Model file for the job. Use its own axes, mm. Face numbers are marked on the shaded views. A direction names the side the tool comes from. Coordinates: 2 decimals unless noted, no trailing zeros. Write each loop counter-clockwise with the first axis right and the second up, starting at its lowest first coordinate (ties: lowest second). Pieces come first, ordered by that corner, then holes. Notation, with made-up numbers: M -18,-9.5 L 0,-9.5 A27 ccw 0,28.5 Z; hole C -36.5,-13 d9. An arc over 180 degrees is marked long. One line per question, with ' | ' between items. Start each with the question number.
(1) Cut at A-A (x = -1415). Write the cut outline in (y, z).
(2) Cut at D-D (x = -1448.5). Write the cut outline in (y, z).
(3) Two-plate mould, pull along X, no slides. Class the marked faces 3, 4 and 5: +X half, -X half, draft (parallel to the pull), parting line (faces both ways), or undercut.
(4) Tool access for the marked faces 1 and 2: list every direction of +Z, -Z, +X, -X, +Y, -Y with a clear straight run to the whole face (end or side of a thin tool).
(5) Cut at B-B (y = 2.2). Write the cut outline in (x, z).
(6) Cut at C-C (z = -991.5). Write the cut outline in (x, y).
(7) Flat gauge pins, fed straight in: pin 1 Ø1.5 at (x, y) = (-1443, 1.5) entering from +Z; pin 2 Ø1 at (y, z) = (1.5, -1005) entering from -X; pin 3 Ø1.5 at (y, z) = (3.5, -992.5) entering from -X. Where does each tip first touch, or does it go through?
(8) Wall check: probe 1 along X at (y, z) = (1.6, -989.75); probe 2 along Z at (x, y) = (-1415, 3.65); probe 3 along Z at (x, y) = (-1415.5, 1.6). Give the ranges that are in metal, low to high.
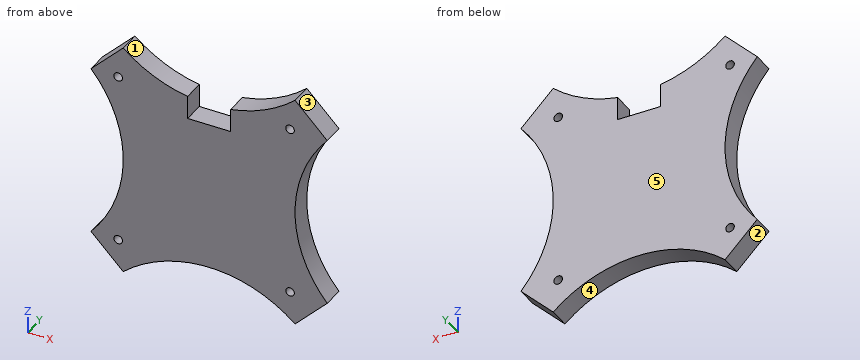
from build123d import *

# Parameters (mm, degrees)
SKETCH1_R           = 1
BOSS_EXTRUDE1_DEPTH = 5


with BuildPart() as part:
    # Sketch1 → Boss-Extrude1 (new body)
    with BuildSketch(Plane(origin=(0, 0, 0), x_dir=(1, 0, 0), z_dir=(0, 1, 0))):
        with BuildLine():
            ThreePointArc((-1438.835902455, 989.336226708), (-1446.828348365, 986.835514311), (-1453.835902334, 982.25))
            Line((-1453.835902334, 982.25), (-1461.335900746, 989.750001588))
            ThreePointArc((-1461.335900746, 989.750001588), (-1453.835896511, 1009.75), (-1461.335892276, 1029.750001588))
            Line((-1461.335892276, 1029.750001588), (-1453.835890688, 1037.25))
            ThreePointArc((-1453.835890688, 1037.25), (-1433.835890688, 1029.75), (-1413.835890688, 1037.25))
            Line((-1413.835890688, 1037.25), (-1406.335890688, 1029.749996824))
            ThreePointArc((-1406.335890688, 1029.749996824), (-1413.835886887, 1009.750002768), (-1406.335890688, 989.750008712))
            Line((-1406.335890688, 989.750008712), (-1413.835902577, 982.25))
            ThreePointArc((-1413.835902577, 982.25), (-1420.843456545, 986.835514311), (-1428.835902455, 989.336226708))
            Line((-1428.835902455, 989.336226708), (-1428.835902455, 989.75))
            Line((-1428.835902455, 989.75), (-1428.835902455, 994.75))
            Line((-1428.835902455, 994.75), (-1433.835902455, 994.75))
            Line((-1433.835902455, 994.75), (-1438.835902455, 994.75))
            Line((-1438.835902455, 994.75), (-1438.835902455, 989.75))
            Line((-1438.835902455, 989.75), (-1438.835902455, 989.336226708))
        make_face()
        with Locations((-1415, 989.75)):
            Circle(SKETCH1_R, mode=Mode.SUBTRACT)
        with Locations((-1455.000010057, 989.75)):
            Circle(SKETCH1_R, mode=Mode.SUBTRACT)
        with Locations((-1415, 1029.75)):
            Circle(SKETCH1_R, mode=Mode.SUBTRACT)
        with Locations((-1455.000001588, 1029.75)):
            Circle(SKETCH1_R, mode=Mode.SUBTRACT)
    extrude(amount=BOSS_EXTRUDE1_DEPTH)


solid = part.part
Filled in:
1) outline: M 0,-1036.28 L 5,-1036.28 L 5,-1030.75 L 0,-1030.75 Z; M 0,-1028.75 L 5,-1028.75 L 5,-990.75 L 0,-990.75 Z; M 0,-988.75 L 5,-988.75 L 5,-983.22 L 0,-983.22 Z
2) outline: M 0,-1033.52 L 5,-1033.52 L 5,-985.98 L 0,-985.98 Z
3) face 3: +X half | face 4: undercut | face 5: draft
4) face 1: +Z, +Y, -Y | face 2: -Z, -X, +Y, -Y
5) outline: M -1461.34,-1029.75 L -1453.84,-1037.25 A30.42 cw -1413.84,-1037.25 L -1406.34,-1029.75 A30.42 cw -1406.34,-989.75 L -1413.84,-982.25 A30.42 cw -1428.84,-989.34 L -1428.84,-994.75 L -1438.84,-994.75 L -1438.84,-989.34 A30.42 cw -1453.84,-982.25 L -1461.34,-989.75 A30.42 cw Z; hole C -1455,-1029.75 d2; hole C -1455,-989.75 d2; hole C -1415,-1029.75 d2; hole C -1415,-989.75 d2
6) outline: M -1459.92,0 L -1438.84,0 L -1438.84,5 L -1459.92,5 Z; M -1428.84,0 L -1407.75,0 L -1407.75,5 L -1428.84,5 Z
7) pin 1: z = -988.09 | pin 2: x = -1454.29 | pin 3: x = -1459.73
8) probe 1: -1461.34 to -1456, -1454 to -1438.84, -1428.84 to -1416, -1414 to -1406.34 | probe 2: -1036.28 to -1030.75, -1028.75 to -990.75, -988.75 to -983.22 | probe 3: -1035.9 to -1030.62, -1028.88 to -990.62, -988.88 to -983.6
